from build123d import *

# Parameters (mm, degrees)
SKETCH_1_W                    = 40
SKETCH_1_H                    = 80
SM_BASE_FLANGE_1_DEPTH        = 3
OTHER_START                   = -3
OTHER_1_DEPTH                 = 3
HOLE_WIZARD_M8_1_D            = 9
HOLE_WIZARD_M8_1_DEPTH        = 12.4
HOLE_WIZARD_M8_1_CSINK_D      = 9.05
HOLE_WIZARD_M8_1_CSINK_ANGLE  = 90
HOLE_WIZARD_M8_1_TIP          = 2.703872786
HOLE_WIZARD_M10_1_D           = 11
HOLE_WIZARD_M10_1_DEPTH       = 12.4
HOLE_WIZARD_M10_1_CSINK_D     = 11.05
HOLE_WIZARD_M10_1_CSINK_ANGLE = 90
HOLE_WIZARD_M10_1_TIP         = 3.304733405


# Read off the part's stored shape, not the designer's step: 断开-边角1
# Sheet-metal steps are written as plain solids
with BuildPart() as part:
    # Sketch 1 → 基体-法兰1 (new body)
    with BuildSketch(Plane.XY):
        Rectangle(SKETCH_1_W, SKETCH_1_H)
    extrude(amount=-SM_BASE_FLANGE_1_DEPTH)

    # Other 1 outline → Other 1 (cut)
    with BuildSketch(Plane.XY.offset(OTHER_START)):
        with BuildLine():
            ThreePointArc((20, -37), (19.121320344, -39.121320344), (17, -40))
            Line((17, -40), (20, -40))
            Line((20, -40), (20, -37))
        make_face()
        with BuildLine():
            Line((-20, -40), (-17, -40))
            ThreePointArc((-17, -40), (-19.121320344, -39.121320344), (-20, -37))
            Line((-20, -37), (-20, -40))
        make_face()
        with BuildLine():
            ThreePointArc((17, 40), (19.121320344, 39.121320344), (20, 37))
            Line((20, 37), (20, 40))
            Line((20, 40), (17, 40))
        make_face()
        with BuildLine():
            Line((-20, 40), (-20, 37))
            ThreePointArc((-20, 37), (-19.121320344, 39.121320344), (-17, 40))
            Line((-17, 40), (-20, 40))
        make_face()
    extrude(amount=OTHER_1_DEPTH, mode=Mode.SUBTRACT)

    # M8 间隙孔1
    with Locations(Plane.XY):
        with Locations((0, 20), (0, -20)):
            CounterSinkHole(HOLE_WIZARD_M8_1_D / 2, HOLE_WIZARD_M8_1_CSINK_D / 2, depth=HOLE_WIZARD_M8_1_DEPTH, counter_sink_angle=HOLE_WIZARD_M8_1_CSINK_ANGLE)
            with Locations((0, 0, -(HOLE_WIZARD_M8_1_DEPTH + HOLE_WIZARD_M8_1_TIP / 2))):  # 118° drill point
                Cone(0, HOLE_WIZARD_M8_1_D / 2, HOLE_WIZARD_M8_1_TIP, mode=Mode.SUBTRACT)

    # M10 间隙孔1
    with Locations(Plane.XY):
        with Locations((0, 0)):
            CounterSinkHole(HOLE_WIZARD_M10_1_D / 2, HOLE_WIZARD_M10_1_CSINK_D / 2, depth=HOLE_WIZARD_M10_1_DEPTH, counter_sink_angle=HOLE_WIZARD_M10_1_CSINK_ANGLE)
            with Locations((0, 0, -(HOLE_WIZARD_M10_1_DEPTH + HOLE_WIZARD_M10_1_TIP / 2))):  # 118° drill point
                Cone(0, HOLE_WIZARD_M10_1_D / 2, HOLE_WIZARD_M10_1_TIP, mode=Mode.SUBTRACT)


solid = part.part
Can you work these out from the model? Positions are in its coordinate system, mm. Give positions to 0.01 mm unless a question says otherwise; leave off trailing zeros. Loops run counter-clockwise (first coordinate to the right, second up) from the corner with the lowest first, then second, coordinate; pieces in that order, holes last. Notation, with made-up numbers: (61, 56.5) -> (102, 56.5) arc R12 cw to (102, 71.5) -> close; hole circle Ø7 at (28.5, 44). An arc over 180 degrees is marked (long way). Write item = value, one per line.
1) Thinking about a two-plate mould opening in Y: for faces 1 (the cylindrical face through (19.14, -39.1, -1.52)), 2 (the cylindrical face through (0.59, -15.54, -1.53)), 3 (the flat face through (0, -8, -3)), which applies, released by +Y, released by -Y, zero draft, split by the parting line, or undercut?
Check result:
face_1 = released by -Y
face_2 = undercut
face_3 = zero draft
2) Will these pins go through, and if not, where does the flat tip stop? pin 1 (7 mm diameter, centred on x = 0, y = -20, fed in from +Z); pin 2 (5 mm diameter, centred on x = 5, y = 25.5, fed in from +Z).
Check result:
pin_1 = through
pin_2 = 0
3) Suppose I cut it at C-C on y = 0. Write out the boundary of the cut face in (x, z) (3 decimals).
Check result:
outline = (-20, -3) -> (-5.5, -3) -> (-5.5, -0.025) -> (-5.525, 0) -> (-20, 0) -> close; (5.5, -3) -> (20, -3) -> (20, 0) -> (5.525, 0) -> (5.5, -0.025) -> close
4) I need wall thicknesses on L1, parallel to Y at x = 0, z = -2.2; L2, parallel to X at y = -20, z = -0.8; L3, parallel to X at y = 17, z = -2.3. Which ranges of each line are inside material? Lowest first, please. Write a range as from..to.
Check result:
L1 = -40..-24.5, -15.5..-5.5, 5.5..15.5, 24.5..40
L2 = -20..-4.5, 4.5..20
L3 = -20..-3.35, 3.35..20
5) Suppose I cut it at B-B on z = -2.3. Write out the boundary of the cut face in (x, y), then the cut area to 3 significant figures.
Check result:
outline = (-20, -37) arc R3 ccw to (-17, -40) -> (17, -40) arc R3 ccw to (20, -37) -> (20, 37) arc R3 ccw to (17, 40) -> (-17, 40) arc R3 ccw to (-20, 37) -> close; hole circle Ø11 at (0, 0); hole circle Ø9 at (0, -20); hole circle Ø9 at (0, 20)
area = 2,970 mm2
6) Suppose I cut it at A-A on x = 0. Write out the boundary of the cut face in (y, z) (3 decimals), then the cut area to 3 significant figures.
Check result:
outline = (-40, -3) -> (-24.5, -3) -> (-24.5, -0.025) -> (-24.525, 0) -> (-40, 0) -> close; (-15.5, -3) -> (-5.5, -3) -> (-5.5, -0.025) -> (-5.525, 0) -> (-15.475, 0) -> (-15.5, -0.025) -> close; (5.5, -3) -> (15.5, -3) -> (15.5, -0.025) -> (15.475, 0) -> (5.525, 0) -> (5.5, -0.025) -> close; (24.5, -3) -> (40, -3) -> (40, 0) -> (24.525, 0) -> (24.5, -0.025) -> close
area = 153 mm2
7) Suppose I cut it at D-D on y = -20. Write out the boundary of the cut face in (x, z) (3 decimals), then the cut area to 3 significant figures.
Check result:
outline = (-20, -3) -> (-4.5, -3) -> (-4.5, -0.025) -> (-4.525, 0) -> (-20, 0) -> close; (4.5, -3) -> (20, -3) -> (20, 0) -> (4.525, 0) -> (4.5, -0.025) -> close
area = 93.0 mm2
